The drawing under review shows one solid part. Ordinate dimensions are in mm from its lowest x, y, z. Coordinates: 2 decimals unless noted, no trailing zeros. Write each loop counter-clockwise with the first axis right and the second up, starting at its lowest first coordinate (ties: lowest second). Pieces come first, ordered by that corner, then holes. Notation, with made-up numbers: M -39.75,-22 L -20.75,-22 A17 cw -20.75,-8 Z; hole C 27,36.25 d3. An arc over 180 degrees is marked long. Write each question's results on one line, items separated by ' | '. Start each with the question number.
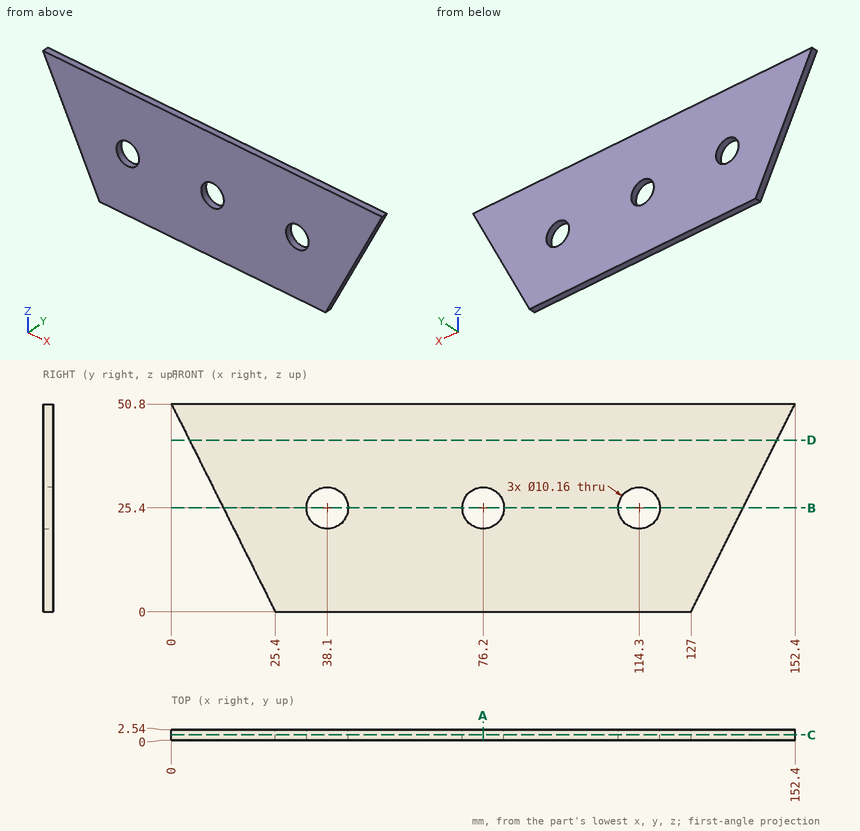
Item 1: Insertion check: pin 1 Ø6 at (x, z) = (114.3, 25.4) entering from -Y. The pin has a flat end and moves straight along its axis. Give the tip position at first contact, or say it passes through.
Item 2: We need section C-C on y = 1.3. State the section outline as (x, z) points, then the cut area to 3 significant figures.
Item 3: We need section D-D on z = 42. State the section outline as (x, y) points.
Item 4: We need section B-B on z = 25.4. State the section outline as (x, y) points.
Item 5: Wall thickness on L1, parallel to X at y = 1, z = 25.4; L2, parallel to X at y = 2.4, z = 21.5; L3, parallel to Z at x = 145, y = 0.2: over which ranges is each line inside the solid? List them lowest first.
Item 6: We need section A-A on x = 76.2. State the section outline as (y, z) points, then the cut area to 3 significant figures.
Answer:
1) pin 1: passes through
2) outline: M 0,50.8 L 25.4,0 L 127,0 L 152.4,50.8 Z; hole C 38.1,25.4 d10.16; hole C 76.2,25.4 d10.16; hole C 114.3,25.4 d10.16 | area: 6,210 mm^2
3) outline: M 4.4,0 L 148,0 L 148,2.54 L 4.4,2.54 Z
4) outline: M 12.7,0 L 33.02,0 L 33.02,2.54 L 12.7,2.54 Z; M 43.18,0 L 71.12,0 L 71.12,2.54 L 43.18,2.54 Z; M 81.28,0 L 109.22,0 L 109.22,2.54 L 81.28,2.54 Z; M 119.38,0 L 139.7,0 L 139.7,2.54 L 119.38,2.54 Z
5) L1: x = 12.7 to 33.02, 43.18 to 71.12, 81.28 to 109.22, 119.38 to 139.7 | L2: x = 14.65 to 34.84, 41.36 to 72.94, 79.46 to 111.04, 117.56 to 137.75 | L3: z = 36 to 50.8
6) outline: M 0,0 L 2.54,0 L 2.54,20.32 L 0,20.32 Z; M 0,30.48 L 2.54,30.48 L 2.54,50.8 L 0,50.8 Z | area: 103 mm^2
